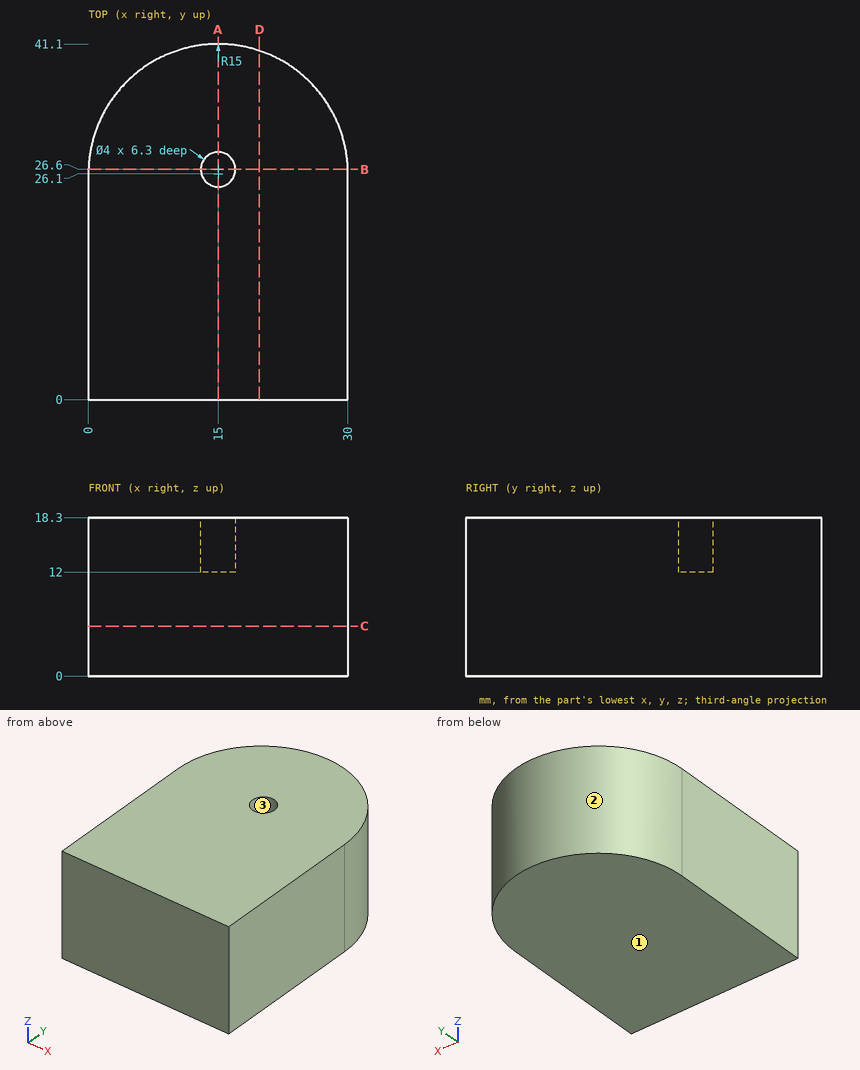
Study the drawing (mm; zero at the part's minimum x, y, z) and answer. Coordinates: 2 decimals unless noted, no trailing zeros. Loops run counter-clockwise (first coordinate to the right, second up) from the corner with the lowest first, then second, coordinate; pieces in that order, holes last. Notation, with made-up numbers: (43, 81.25) -> (54, 81.25) arc R27 cw to (54, 104.25) -> close; hole circle Ø8 at (-25.5, 26.25). An arc over 180 degrees is marked (long way). Write each question's results on one line, items separated by ' | '. Start each with the question number.
1) A flat-ended cylindrical pin translates along its axis: P1, Ø4, axis at y = 31.5, z = 4, coming from the -X side. Find the tip coordinate at first contact, or state that the pin passes through.
2) Find section A-A on x = 15. Determine the outline of the cut face in (y, z), then the cut area to 3 significant figures.
3) Consider line 1 along Y through (x, z) = (15, 14); line 2 along Z through (x, y) = (13.5, 25.5); line 3 along X through (y, z) = (35, 15.5). Determine where each line is inside the solid, lowest interval first.
4) Find section B-B on y = 26.6. Determine the outline of the cut face in (x, z).
5) The mould has two halves that part along Y. Classify the marked faces 1, 2 and 3: pulls with the +Y half, pulls with the -Y half, needs draft (parallel to the pull), parting line crosses it, or undercut.
6) Find section D-D on x = 19.75. Determine the outline of the cut face in (y, z).
7) Find section C-C on z = 5.75. Determine the outline of the cut face in (x, y), then the cut area to 3 significant figures.
Response values:
1) P1: stops at x = 0.39
2) outline: (0, 0) -> (41.1, 0) -> (41.1, 18.3) -> (28.6, 18.3) -> (28.6, 12) -> (24.6, 12) -> (24.6, 18.3) -> (0, 18.3) -> close | area: 727 mm^2
3) line 1: y = 0 to 24.6, 28.6 to 41.1 | line 2: z = 0 to 12 | line 3: x = 2.93 to 27.07
4) outline: (0.01, 0) -> (29.99, 0) -> (29.99, 18.3) -> (17, 18.3) -> (17, 12) -> (13, 12) -> (13, 18.3) -> (0.01, 18.3) -> close
5) face 1: needs draft | face 2: pulls with the +Y half | face 3: undercut
6) outline: (0, 0) -> (40.33, 0) -> (40.33, 18.3) -> (0, 18.3) -> close
7) outline: (0, 0) -> (30, 0) -> (30, 26.1) arc R15 ccw to (0, 26.1) -> close | area: 1,140 mm^2
